Build history of the part. All positions in model axes, mm. Face numbers are marked on the shaded views. A direction names the side the tool comes from. Give positions to 0.01 mm unless a question says otherwise; leave off trailing zeros. Order: outer loops, then holes, each group sorted by start corner. A loop starts at its lowest first (then second) coordinate and runs counter-clockwise, first axis right, second up. Notation, with made-up numbers: (61, -17) -> (85, -17) arc R10 cw to (85, -11) -> close; hole circle Ø9 at (8, 40.5). An arc over 180 degrees is marked (long way). One line per item, written item: value. Start each with the question number.
(1) Saw through at C-C on z = 42. Give the cut face in (x, y).
(2) Saw through at A-A on y = 0. Give the cut face in (x, z).
(3) Saw through at B-B on x = 42.5. Give the cut face in (y, z).
(4) Pin check, flat tips, straight feed: pin 1 (1.5 mm diameter, centred on y = 5.5, z = 41.5, fed in from -X); pin 2 (8.5 mm diameter, centred on x = -104.79, y = -60.5, fed in from -Z); pin 3 (6 mm diameter, centred on x = -87, z = 157, fed in from +Y). Stop position of each tip, or through.
(5) Saw through at D-D on x = -116.5. Give the cut face in (y, z), plus the area to 3 significant figures.
(6) Which spindle directions (+Z, -Z, +X, -X, +Y, -Y) get a long thin tool onto all of the face, cutting with end or side? Do the marked faces 1 and 2. Say none if no direction does.
(7) Probe line 1 (X direction, y = 60, z = 190); line 2 (Z direction, x = 108.5, y = 31.5); line 3 (X direction, y = 31.5, z = 91). List the from-to ranges inside material, lowest first.
```python
from build123d import *

# Parameters (mm, degrees)
SKETCH1_R           = 106
SKETCH1_R_2         = 101
BOSS_EXTRUDE1_DEPTH = 200
BOSS_EXTRUDE3_START = -20
SKETCH3_R           = 136
SKETCH3_R_2         = 106
BOSS_EXTRUDE3_DEPTH = 20
SKETCH5_R           = 111.5
SKETCH5_R_2         = 108.5
CUT_EXTRUDE1_DEPTH  = 4
SKETCH4_R           = 3.3
CUT_EXTRUDE2_DEPTH  = 33
CIRPATTERN1_COUNT   = 6


with BuildPart() as part:
    # Sketch1 → Boss-Extrude1 (new body)
    with BuildSketch(Plane.XY):
        Circle(SKETCH1_R)
        Circle(SKETCH1_R_2, mode=Mode.SUBTRACT)
    extrude(amount=BOSS_EXTRUDE1_DEPTH)

    # Sketch3 → Boss-Extrude3 (add)
    with BuildSketch(Plane.XY.offset(200).offset(BOSS_EXTRUDE3_START)):
        Circle(SKETCH3_R)
        Circle(SKETCH3_R_2, mode=Mode.SUBTRACT)
    extrude(amount=BOSS_EXTRUDE3_DEPTH)

    # Sketch5 → Cut-Extrude1 (cut)
    with BuildSketch(Plane.XY.offset(200)):
        Circle(SKETCH5_R)
        Circle(SKETCH5_R_2, mode=Mode.SUBTRACT)
    extrude(amount=-CUT_EXTRUDE1_DEPTH, mode=Mode.SUBTRACT)

    # Sketch4 → Cut-Extrude2 (cut)
    with BuildSketch(Plane.XY.offset(200)):
        with Locations((0, 121)):
            Circle(SKETCH4_R)
    cut_extrude2 = extrude(amount=-CUT_EXTRUDE2_DEPTH, mode=Mode.SUBTRACT)

    # CirPattern1: Cut-Extrude2 ×6 about axis
    cirpattern1_axis = Axis((0, 0, 0), (0, 0, 1))
    for i in range(1, CIRPATTERN1_COUNT):
        add(cut_extrude2.rotate(cirpattern1_axis, i * 360 / CIRPATTERN1_COUNT), mode=Mode.SUBTRACT)


solid = part.part
```
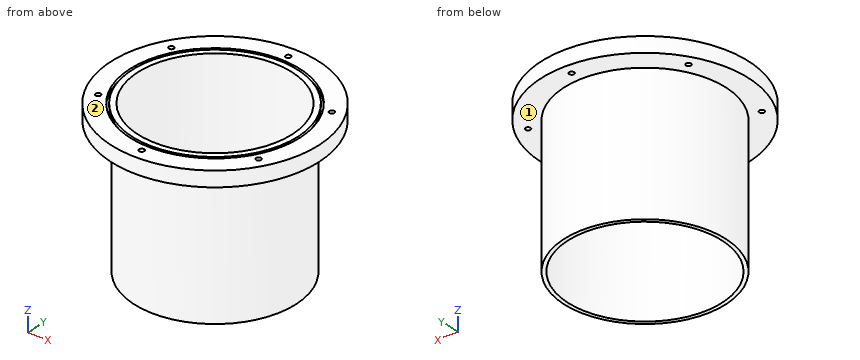
Results below:
1. outline: circle Ø212 at (0, 0); hole circle Ø202 at (0, 0)
2. outline: (-136, 180) -> (-106, 180) -> (-106, 0) -> (-101, 0) -> (-101, 200) -> (-108.5, 200) -> (-108.5, 196) -> (-111.5, 196) -> (-111.5, 200) -> (-136, 200) -> close; (101, 0) -> (106, 0) -> (106, 180) -> (136, 180) -> (136, 200) -> (111.5, 200) -> (111.5, 196) -> (108.5, 196) -> (108.5, 200) -> (101, 200) -> close
3. outline: (-129.19, 180) -> (-97.11, 180) -> (-97.11, 0) -> (-91.62, 0) -> (-91.62, 200) -> (-99.83, 200) -> (-99.83, 196) -> (-103.08, 196) -> (-103.08, 200) -> (-129.19, 200) -> close; (91.62, 0) -> (97.11, 0) -> (97.11, 180) -> (129.19, 180) -> (129.19, 200) -> (103.08, 200) -> (103.08, 196) -> (99.83, 196) -> (99.83, 200) -> (91.62, 200) -> close
4. pin 1: stops at x = -105.89
4. pin 2: stops at z = 180
4. pin 3: stops at y = 64.65
5. outline: (-70.17, 180) -> (70.17, 180) -> (70.17, 200) -> (-70.17, 200) -> close
5. area: 2,810 mm²
6. face 1: -Z
6. face 2: +Z, +X, -X, +Y, -Y
7. line 1: x = -122.05 to -108.05, -101.53 to -81.25, 81.25 to 101.53, 108.05 to 122.05
7. line 2: z = 180 to 200
7. line 3: x = -101.21 to -95.96, 95.96 to 101.21
